Can you work these out from the model? Positions are in its coordinate system, mm. A direction names the side the tool comes from. Round coordinates to 2 decimals unless told otherwise and drop trailing zeros. Write each loop counter-clockwise with the first axis right and the second up, starting at its lowest first coordinate (ties: lowest second). Pieces come first, ordered by that corner, then holes. Notation, with made-up numbers: (59, 21) -> (69, 21) arc R23 cw to (69, 29) -> close; hole circle Ø3 at (61.25, -34.5). An arc over 180 degrees is marked (long way). Write item = value, one per line. Start each with the question number.
1) For faces 4 (the face through (-3.86, -7.64, 5.04)), 5 (the face through (5.08, -3, 0)), 6 (the face through (0, -3, -2.54)), which set-ups out of +Z, -Z, +X, -X, +Y, -Y let a thin tool reach every point of the face, with its end or its side?
2) If I drill on line 1 (X direction, y = -5.5, z = 1.25); line 2 (Y direction, x = 0.5, z = 1.5), over which ranges is the centre line in solid material (lowest first)?
3) Thinking about a two-plate mould opening in X: for faces 1 (the face through (0, -3, 2.54)), 2 (the face through (0, -3, 5.08)), 3 (the face through (-5.08, -3, 0)), which applies, +X half, -X half, draft (parallel to the pull), parting line (faces both ways), or undercut?
4) I'm going to push flat-ended pins straight in: pin 1 (4 mm diameter, centred on y = -8.5, z = 3.5, fed in from -X); pin 2 (1.3 mm diameter, centred on x = 0.5, y = -4, fed in from +Z); pin 3 (1 mm diameter, centred on y = 1, z = -1, fed in from +X). Where does each tip first touch, or does it pass through?
5) Imagine slicing it at A-A, the plane y = -8. Please give me the cut outline in (x, z), then the cut area to 3 significant figures.
from build123d import *

# Parameters (mm, degrees)
SKETCH1_W             = 6.35
SKETCH1_H             = 3.175
DOMEY_TOP_FACE_RADIUS = 6.35
DOMEY_TOP_HEIGHT      = 2.54
ONE_LEG_DEPTH         = 6.35
ALL_LEGS_COUNT        = 4
BASE_START            = 2.54
SKETCH3_R             = 6.35
BASE_DEPTH            = 2.54


with BuildPart() as part:
    # Sketch1 → button top (revolve)
    with BuildSketch(Plane.XY, mode=Mode.PRIVATE) as button_top_sk:
        with Locations((-3.175, 1.5875)):
            Rectangle(SKETCH1_W, SKETCH1_H)
    revolve(button_top_sk.sketch.rotate(Axis((0, 0, 0), (0, 1, 0)), 270), axis=Axis((0, 0, 0), (0, 1, 0)))

    # domey top: a dome of height H over a round flat face of radius A is a cap of a sphere of radius (A * A + H * H) / (2 * H)
    domey_top_r = (DOMEY_TOP_FACE_RADIUS * DOMEY_TOP_FACE_RADIUS + DOMEY_TOP_HEIGHT * DOMEY_TOP_HEIGHT) / (2 * DOMEY_TOP_HEIGHT)
    domey_top_base = Plane((0, 3.175, 0), z_dir=(0, 1, 0))
    with Locations(domey_top_base.offset(DOMEY_TOP_HEIGHT - domey_top_r)):
        domey_top_ball = Sphere(domey_top_r, mode=Mode.PRIVATE)
    add(split(domey_top_ball, bisect_by=domey_top_base, keep=Keep.TOP, mode=Mode.PRIVATE))

    # Sketch2 → one leg (add)
    with BuildSketch(Plane.XZ):
        with BuildLine():
            Line((-1.27, -2.54), (1.27, -2.54))
            ThreePointArc((1.27, -2.54), (2.54, -3.81), (1.27, -5.08))
            Line((1.27, -5.08), (-1.27, -5.08))
            ThreePointArc((-1.27, -5.08), (-2.54, -3.81), (-1.27, -2.54))
        make_face()
    one_leg = extrude(amount=ONE_LEG_DEPTH)

    # all legs: one leg ×4 about axis
    all_legs_axis = Axis((0, 0, 0), (0, 1, 0))
    for i in range(1, ALL_LEGS_COUNT):
        add(one_leg.rotate(all_legs_axis, i * 360 / ALL_LEGS_COUNT))

    # Sketch3 → base (add)
    with BuildSketch(Plane.XZ.offset(6.35).offset(BASE_START)):
        with Locations(Location((0, 0, 0), (0, 0, 270))):
            Circle(SKETCH3_R)
    extrude(amount=-BASE_DEPTH)

    # Sketch6 → Revolve2 (revolve)
    with BuildSketch(Plane(origin=(0, 0, 0), x_dir=(0, 0, -1), z_dir=(1, 0, 0))):
        with BuildLine():
            Line((0, -8.89), (0, -11.938))
            add(Edge.make_bspline(
                [(0, -11.938), (2.963289741, -11.938), (5.038193669, -11.554158935), (6.35, -8.89)],
                knots=[0, 0, 0, 0, 1, 1, 1, 1], degree=3))
            Line((6.35, -8.89), (0, -8.89))
        make_face()
    revolve(axis=Axis((0, -8.89, 0), (0, -1, 0)))


solid = part.part
Reported:
q1.face_4 = +Y, -Y
q1.face_5 = +Z, -Z, +X
q1.face_6 = none
q2.line_1 = -5.08 to -2.54, 2.54 to 5.08
q2.line_2 = -11.88 to -6.35, 0 to 5.58
q3.face_1 = undercut
q3.face_2 = draft
q3.face_3 = -X half
q4.pin_1 = -6.17
q4.pin_2 = 5.08
q4.pin_3 = 6.33
q5.outline = circle Ø12.7 at (0, 0)
q5.area = 127 mm²
